Here's how the part is built. I have some questions about the finished solid (model axes, mm). Face numbers are marked on the shaded views. A direction names the side the tool comes from. Give positions to 0.01 mm unless a question says otherwise; leave off trailing zeros. Order: outer loops, then holes, each group sorted by start corner. A loop starts at its lowest first (then second) coordinate and runs counter-clockwise, first axis right, second up. Notation, with made-up numbers: (-22, 75.25) - (-12, 75.25) arc R20 ccw to (-12, 84.25) - close; hole circle Ø3 at (4, 86.25). An arc over 180 degrees is marked (long way). One line per question, with ' | ' between items.
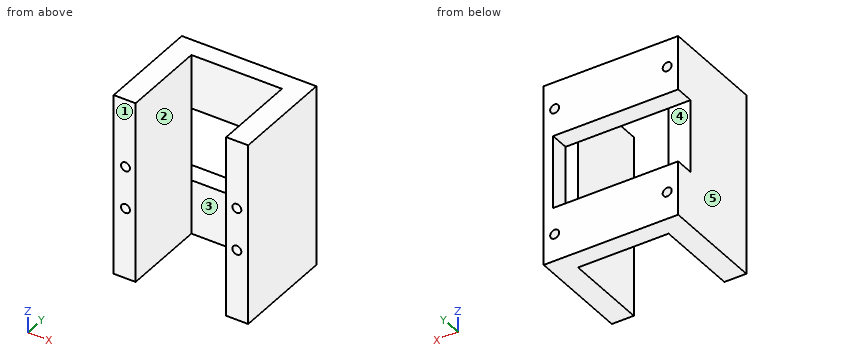
from build123d import *

# Parameters (mm, degrees)
SKETCH1_W           = 57
SKETCH1_H           = 37
BOSS_EXTRUDE1_DEPTH = 44
SKETCH2_W           = 38.4
SKETCH2_H           = 36
CUT_EXTRUDE1_DEPTH  = 47
SKETCH4_R           = 1.9
CUT_EXTRUDE3_DEPTH  = 30
BOSS_EXTRUDE2_DEPTH = 20
BOSS_EXTRUDE3_DEPTH = 20
SKETCH7_W           = 53
SKETCH7_H           = 31
CUT_EXTRUDE4_DEPTH  = 8
SKETCH8_R           = 1.9
CUT_EXTRUDE5_DEPTH  = 25


with BuildPart() as part:
    # Sketch1 → Boss-Extrude1 (new body)
    with BuildSketch(Plane(origin=(0, 0, 0), x_dir=(1, 0, 0), z_dir=(0, 1, 0))):
        Rectangle(SKETCH1_W, SKETCH1_H)
    extrude(amount=BOSS_EXTRUDE1_DEPTH)

    # Sketch2 → Cut-Extrude1 (cut)
    with BuildSketch(Plane.XY.offset(18.5)):
        with Locations((0, 18)):
            Rectangle(SKETCH2_W, SKETCH2_H)
    extrude(amount=-CUT_EXTRUDE1_DEPTH, mode=Mode.SUBTRACT)

    # Sketch4 → Cut-Extrude3 (cut)
    with BuildSketch(Plane.XZ):
        with Locations(Location((23.704806449, 9.5, 0), (0, 0, 270))):
            Circle(SKETCH4_R)
        with Locations(Location((23.704806449, -8.5, 0), (0, 0, 270))):
            Circle(SKETCH4_R)
        with Locations(Location((-23.5, 9.5, 0), (0, 0, 270))):
            Circle(SKETCH4_R)
        with Locations(Location((-23.5, -8.5, 0), (0, 0, 270))):
            Circle(SKETCH4_R)
    extrude(amount=-CUT_EXTRUDE3_DEPTH, mode=Mode.SUBTRACT)

    # Sketch5 → Boss-Extrude2 (add)
    with BuildSketch(Plane(origin=(0, 0, -18.5), x_dir=(-1, 0, 0), z_dir=(0, 0, -1))):
        Polygon((-19.2, 36), (19.2, 36), (19.2, 0), (28.5, 0), (28.5, 44), (-28.5, 44), (-28.5, 0), (-19.2, 0), align=None)
    extrude(amount=BOSS_EXTRUDE2_DEPTH)

    # Sketch6 → Boss-Extrude3 (add)
    with BuildSketch(Plane.XY.offset(18.5)):
        Polygon((-28.5, 0), (-19.2, 0), (-19.2, 36), (19.2, 36), (19.2, 0), (28.5, 0), (28.5, 44), (-28.5, 44), align=None)
    extrude(amount=BOSS_EXTRUDE3_DEPTH)

    # Sketch7 → Cut-Extrude4 (cut)
    with BuildSketch(Plane(origin=(0, 44, 0), x_dir=(1, 0, 0), z_dir=(0, 1, 0))):
        with Locations((-2, 0)):
            Rectangle(SKETCH7_W, SKETCH7_H)
    extrude(amount=-CUT_EXTRUDE4_DEPTH, mode=Mode.SUBTRACT)

    # Sketch8 → Cut-Extrude5 (cut)
    with BuildSketch(Plane(origin=(0, 44, 0), x_dir=(1, 0, 0), z_dir=(0, 1, 0))):
        with Locations(Location((23.85, -27, 0), (0, 0, 270))):
            Circle(SKETCH8_R)
        with Locations(Location((-23.85, -27, 0), (0, 0, 270))):
            Circle(SKETCH8_R)
        with Locations(Location((-23.85, 27, 0), (0, 0, 270))):
            Circle(SKETCH8_R)
        with Locations(Location((23.85, 27, 0), (0, 0, 270))):
            Circle(SKETCH8_R)
    extrude(amount=-CUT_EXTRUDE5_DEPTH, mode=Mode.SUBTRACT)


solid = part.part
1) Please list where these lines run through material, in increasing order: L1, parallel to X at y = 29, z = -27; L2, parallel to X at y = 37, z = -27; L3, parallel to X at y = 31, z = -17.5.
Model answer:
L1: x = -28.5 to -25.75, -21.95 to -19.2, 19.2 to 21.95, 25.75 to 28.5 | L2: x = -28.5 to -25.75, -21.95 to 21.95, 25.75 to 28.5 | L3: x = -28.5 to -19.2, 19.2 to 28.5
2) I want a section at C-C (x = -7.5). List the corners of the cut face in (y, z) for me.
Model answer:
outline: (36, -38.5) - (44, -38.5) - (44, -15.5) - (36, -15.5) - close; (36, 15.5) - (44, 15.5) - (44, 38.5) - (36, 38.5) - close
3) I want a section at A-A (y = 31.5). List the corners of the cut face in (x, z) for me, plus the area to 3 significant figures.
Model answer:
outline: (-28.5, -38.5) - (-19.2, -38.5) - (-19.2, 38.5) - (-28.5, 38.5) - close; (19.2, -38.5) - (28.5, -38.5) - (28.5, 38.5) - (19.2, 38.5) - close; hole circle Ø3.8 at (-23.85, -27); hole circle Ø3.8 at (-23.85, 27); hole circle Ø3.8 at (23.85, -27); hole circle Ø3.8 at (23.85, 27) | area: 1,390 mm2
4) I want a section at D-D (z = 18). List the corners of the cut face in (x, y) for me, plus the area to 3 significant figures.
Model answer:
outline: (-28.5, 0) - (-19.2, 0) - (-19.2, 36) - (19.2, 36) - (19.2, 0) - (28.5, 0) - (28.5, 44) - (-28.5, 44) - close | area: 1,130 mm2
5) On a 3-axis mill with a long thin cutter (end or side, diameter ignored), from which of +Z, -Z, +X, -X, +Y, -Y can I reach the whole of each face in a straight line? I mean the marked faces 1 and 2. Say none if no direction works.
Model answer:
face 1: +Z, -Z, +X, -X, -Y | face 2: +Z, -Z, -Y
6) Thinking about a two-plate mould opening in X: for the marked faces 3, 4 and 5, which applies, +X half, -X half, draft (parallel to the pull), parting line (faces both ways), or undercut?
Model answer:
face 3: undercut | face 4: draft | face 5: -X half
7) I want a section at B-B (z = 6.5). List the corners of the cut face in (x, y) for me, plus the area to 3 significant figures.
Model answer:
outline: (-28.5, 0) - (-19.2, 0) - (-19.2, 36) - (-28.5, 36) - close; (19.2, 0) - (28.5, 0) - (28.5, 44) - (24.5, 44) - (24.5, 36) - (19.2, 36) - close | area: 702 mm2
8) I'm going to push flat-ended pins straight in: P1, Ø1.1, axis at x = 23, z = -27, coming from the +Y side; P2, Ø1.1, axis at x = -23.5, z = -9, coming from the -Y side; P3, Ø11.5, axis at x = 7, z = 28, coming from the -Y side. Where does each tip first touch, or does it pass through?
Model answer:
P1: stops at y = 19 | P2: stops at y = 30 | P3: stops at y = 36
